Autodesk Inventor part; units mm, degrees
ref_plane "Work Plane1" through (183.8728, 183.8728, 7.5) normal (0.7071, -0.7071, 0) x (0, 0, -1)
ref_plane "YZ Plane" through (0, 0, 0) normal (1, 0, 0) x (0, 1, 0)
ref_plane "XZ Plane" through (0, 0, 0) normal (0, 1, 0) x (-1, 0, 0)
sketch "Sketch1" plane through (0, 0, 0) normal (0, 0, 1) x (1, 0, 0)
  line L0 (202, 202) -> (202, 0) construction
  line L1 (0, 202) -> (202, 202) construction
  arc A0 (206.2012, 222.0831) -> (193.0425, 222.9456) centre (199.1301, 215.012) ccw
  arc A1 (222.9456, 193.0425) -> (222.0831, 206.2012) centre (215.012, 199.1301) ccw
  line L2 (206.2012, 222.0831) -> (222.0831, 206.2012)
  line L3 (193.0425, 222.9456) -> (165.7457, 202)
  line L4 (202, 165.7457) -> (222.9456, 193.0425)
  line L5 (165.7457, 202) -> (202, 165.7457)
  point P0 (0, 0)
extrude "Extrusion3" add sketch "Sketch1" along normal blind 19
sketch "Sketch3" plane through (0, 0, 19) normal (0, 0, 1) x (1, 0, 0)
  line L0 (165.7457, 202) -> (202, 202)
  line L1 (202, 202) -> (202, 165.7457)
  line L2 (165.7457, 202) -> (202, 165.7457)
  point P0 (0, 0)
extrude "Extrusion4" cut sketch "Sketch3" against normal blind 11.5
sketch "Sketch5" plane through (0, 0, 19) normal (0, 0, 1) x (1, 0, 0)
  line L0 (222.0831, 206.2012) -> (206.2012, 222.0831) construction
  line L1 (214.1421, 214.1421) -> (134.2284, 134.2284) construction
  line L2 (202, 165.7457) -> (165.7457, 202) construction
  circle A0 centre (190.9439, 190.9439) radius 6
  point P0 (0, 0)
  dimension "d25" = 12
  dimension "d26" = 10
extrude "Extrusion6" cut sketch "Sketch5" against normal through all
sketch "Sketch6" plane through (0, 0, 19) normal (0, 0, 1) x (1, 0, 0)
  circle A0 centre (202, 202) radius 2.75
  point P0 (0, 0)
  dimension "d27" = 5.5
extrude "Extrusion7" cut sketch "Sketch6" against normal through all
sketch "Sketch7" plane through (0, 0, 19) normal (0, 0, 1) x (1, 0, 0)
  arc A0 (202, 199.25) -> (199.25, 202) centre (202, 202) ccw construction
  circle A1 centre (202, 202) radius 16.75
  point P0 (0, 0)
  dimension "d30" = 33.5
extrude "Extrusion8" cut sketch "Sketch7" against normal blind 9
sketch "Sketch8" plane through (0, 0, 19) normal (0, 0, 1) x (1, 0, 0)
  line L0 (202, 185.25) -> (202, 165.7457) construction
  circle A0 centre (190.9439, 190.9439) radius 6 construction
  line L1 (202, 165.7457) -> (165.7457, 202) construction
  line L2 (163.0953, 218.7925) -> (219.2426, 162.6452) construction
  circle A1 centre (202, 179.8878) radius 1.65
  point P0 (0, 0)
  dimension "d33" = 3.3
extrude "Extrusion9" cut sketch "Sketch8" against normal through all
sketch "Sketch9" plane through (0, 0, 19) normal (0, 0, 1) x (1, 0, 0)
  arc A0 (202, 178.2378) -> (202, 181.5378) centre (202, 179.8878) ccw construction
  circle A1 centre (202, 179.8878) radius 3.25
  point P0 (0, 0)
  dimension "d36" = 6.5
extrude "Extrusion10" cut sketch "Sketch9" against normal blind 14
ref_plane "Work Plane1" through (183.8728, 183.8728, 7.5) normal (0.7071, -0.7071, 0) x (0, 0, -1)
mirror "Mirror1" about plane through (183.8728, 183.8728, 7.5) normal (0.7071, -0.7071, 0) of "Extrusion9", "Extrusion10"
fillet "Fillet6" radius 2 4 edges at (165.7457, 202, 13.25) (165.7457, 202, 3.75) (202, 165.7457, 13.25) (202, 165.7457, 3.75)
sketch "Sketch10" plane through (0, 0, 10) normal (0, 0, 1) x (1, 0, 0)
  line L0 (202, 185.25) -> (202, 199.25)
  arc A0 (202, 185.25) -> (185.25, 202) centre (202, 202) ccw
  line L1 (199.25, 202) -> (185.25, 202)
  arc A1 (202, 199.25) -> (199.25, 202) centre (202, 202) ccw
  point P0 (0, 0)
properties part number "leveling clip"
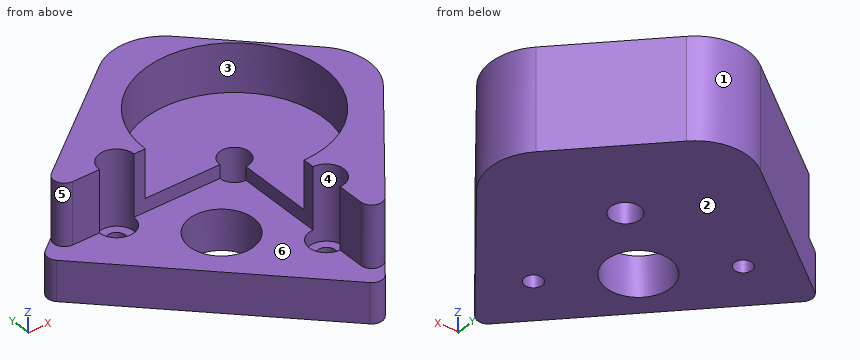
Design review of the part built by this model. Coordinates are the model's own, in mm. Face numbers are marked on the shaded views. A direction names the side the tool comes from. Give positions to 0.01 mm unless a question says otherwise; leave off trailing zeros. Loops run counter-clockwise (first coordinate to the right, second up) from the corner with the lowest first, then second, coordinate; pieces in that order, holes last. Notation, with made-up numbers: M -18.75,85 L -9.75,85 A34 ccw -9.75,120 Z; hole C 37.25,27.25 d10. An arc over 180 degrees is marked long. Return JSON: item names as keys, results as strings. Group by question number.
Item 1: We need section D-D (x = 214). Give the boundary of the cut face in (y, z), and give its area (3 significant figures).
Item 2: We need section C-C (y = 211.5). Give the boundary of the cut face in (x, z).
Item 3: Mouldability with a two-part tool opening along Y and no side actions: class the marked faces 1, 2 and 3 as released by +Y, released by -Y, zero draft, split by the parting line, or undercut.
Item 4: Insertion check: pin 1 Ø2 at (x, y) = (178.5, 200.5) entering from +Z; pin 2 Ø10 at (x, z) = (189.5, 17) entering from +Y; pin 3 Ø4 at (x, z) = (174.5, 13) entering from -Y. Each pin has a flat end and moves straight along its axis. Give the tip position at first contact, or say it passes through.
Item 5: For probe 1 along X at (y, z) = (202, 1.95); probe 2 along Y at (x, z) = (204, 11.25), list the stretches that pass through material, from the lowest coordinate up.
Item 6: We need section A-A (y = 190). Give the boundary of the cut face in (x, z), and give its area (3 significant figures).
Item 7: We need section B-B (z = 6.75). Give the number of separate pieces and of enclosed holes in the cut face, and give its area (3 significant figures).
Item 8: Tool access review of the marked faces 4, 5 and 6: name each direction out of +Z, -Z, +X, -X, +Y, -Y from which nothing blocks a thin tool from reaching the whole face with its end or side.
Output:
{
 "1": {"outline": "M 181.38,0 L 214.28,0 L 214.28,19 L 213.69,19 L 213.69,10 L 190.31,10 L 190.31,19 L 181.38,19 Z", "area": "415 mm^2"},
 "2": {"outline": "M 178.13,0 L 216.78,0 L 216.78,19 L 215.8,19 L 215.8,10 L 188.2,10 L 188.2,19 L 178.13,19 Z"},
 "3": {"face 1": "released by +Y", "face 2": "zero draft", "face 3": "undercut"},
 "4": {"pin 1": "stops at z = 5", "pin 2": "stops at y = 223.88", "pin 3": "stops at y = 202"},
 "5": {"probe 1": "x = 166.78 to 178.24, 181.54 to 199.25, 204.75 to 224.59", "probe 2": "y = 169.64 to 177.33, 182.45 to 185.37, 218.63 to 223.75"},
 "6": {"outline": "M 177.75,0 L 185.02,0 L 185.02,7.5 L 177.75,7.5 Z; M 196.87,0 L 220.61,0 L 220.61,19 L 213.69,19 L 213.69,10 L 202,10 L 202,7.5 L 196.87,7.5 Z", "area": "341 mm^2"},
 "7": {"separate pieces": "1", "enclosed holes": "4", "area": "1,720 mm^2"},
 "8": {"face 4": "+Z", "face 5": "+Z, -X", "face 6": "+Z, -X, -Y"}
}
